from build123d import *

# Parameters (mm, degrees)
BOSS_EXTRUDE1_DEPTH      = 10
BOSS_EXTRUDE1_DEPTH_BACK = 0.01
SKETCH3_W                = 38
SKETCH3_H                = 54
CUT_EXTRUDE1_DEPTH       = 3
SKETCH5_W                = 38
SKETCH5_H                = 54
CUT_EXTRUDE3_DEPTH       = 3
SKETCH7_W                = 169
SKETCH7_H                = 58
CUT_EXTRUDE4_DEPTH       = 261.116514656
SKETCH15_W               = 20
SKETCH15_H               = 50
BOSS_EXTRUDE3_DEPTH      = 20.3
SKETCH18_W               = 47.4
SKETCH18_H               = 47.4
CUT_EXTRUDE18_DEPTH      = 261.715344958
SKETCH21_R               = 9
CUT_EXTRUDE21_DEPTH      = 20
SKETCH28_W               = 4.75290021
SKETCH28_H               = 9.947843747
BOSS_EXTRUDE6_DEPTH      = 115.870057685
SKETCH30_W               = 14.12
SKETCH30_H               = 25
CUT_EXTRUDE25_DEPTH      = 4.5
SKETCH33_R               = 1.55
CUT_EXTRUDE26_DEPTH      = 10.01
SKETCH36_W               = 38
SKETCH36_H               = 2
BOSS_EXTRUDE7_DEPTH      = 37
SKETCH39_R               = 6
SKETCH39_R_2             = 1.55
CUT_EXTRUDE28_DEPTH      = 2
SKETCH42_R               = 6
SKETCH42_R_2             = 1.55
CUT_EXTRUDE29_DEPTH      = 2


with BuildPart() as part:
    # Sketch1 → Boss-Extrude1 (new, two sides: drawn at the far end of the back side and taken through both)
    with BuildSketch(Plane.XY.offset(-BOSS_EXTRUDE1_DEPTH_BACK)):
        with BuildLine():
            Line((0, 0), (0, -37))
            Line((0, -37), (60, -37))
            Line((60, -37), (60, -52))
            Line((60, -52), (33.129942315, -78.870057685))
            Line((33.129942315, -78.870057685), (-55.850057685, -78.870057685))
            ThreePointArc((-55.850057685, -78.870057685), (-169.614041234, -90.257166815), (-239.999947532, -0.158696229))
            ThreePointArc((-239.999947532, -0.158696229), (-169.748285548, 90.207490359), (-55.850057685, 78.870057685))
            Line((-55.850057685, 78.870057685), (33.129942315, 78.870057685))
            Line((33.129942315, 78.870057685), (60, 52))
            Line((60, 52), (60, 37))
            Line((60, 37), (0, 37))
            Line((0, 37), (0, 0))
        make_face()
    extrude(amount=BOSS_EXTRUDE1_DEPTH + BOSS_EXTRUDE1_DEPTH_BACK)

    # Sketch3 → Cut-Extrude1 (cut)
    with BuildSketch(Plane.XY.offset(10)):
        with Locations((-19, 51.870057685)):
            Rectangle(SKETCH3_W, SKETCH3_H)
    extrude(amount=-CUT_EXTRUDE1_DEPTH, mode=Mode.SUBTRACT)

    # Sketch5 → Cut-Extrude3 (cut)
    with BuildSketch(Plane.XY.offset(10)):
        with Locations((-19, -51.870057685)):
            Rectangle(SKETCH5_W, SKETCH5_H)
    extrude(amount=-CUT_EXTRUDE3_DEPTH, mode=Mode.SUBTRACT)

    # Sketch7 → Cut-Extrude4 (cut, through all)
    with BuildSketch(Plane.XY.offset(10)):
        with Locations((-128.91309413, -19.94383898)):
            Rectangle(SKETCH7_W, SKETCH7_H)
    extrude(amount=-CUT_EXTRUDE4_DEPTH, mode=Mode.SUBTRACT)

    # Sketch15 → Boss-Extrude3 (add)
    with BuildSketch(Plane.XY.offset(10)):
        with Locations((-10, 0.20156489)):
            Rectangle(SKETCH15_W, SKETCH15_H)
    extrude(amount=BOSS_EXTRUDE3_DEPTH)

    # Sketch18 → Cut-Extrude18 (cut, through all)
    with BuildSketch(Plane.XY.offset(10)):
        with Locations((-80.42454895, 45.3)):
            Rectangle(SKETCH18_W, SKETCH18_H)
    extrude(amount=-CUT_EXTRUDE18_DEPTH, mode=Mode.SUBTRACT)

    # Sketch21 → Cut-Extrude21 (cut)
    with BuildSketch(Plane(origin=(0, 0, 0), x_dir=(0, 0, -1), z_dir=(1, 0, 0))):
        with Locations((-19.36187505, 12.37175029)):
            Circle(SKETCH21_R)
        with Locations((-19.26539558, -14.62824971)):
            Circle(SKETCH21_R)
        with BuildLine():
            Line((-9.491579533, 2.276446619), (-9.557448357, -4.178698144))
            ThreePointArc((-9.557448357, -4.178698144), (-12.081396215, -6.651657156), (-14.554355227, -4.127709299))
            Line((-14.554355227, -4.127709299), (-14.488486403, 2.327435464))
            ThreePointArc((-14.488486403, 2.327435464), (-11.964538545, 4.800394476), (-9.491579533, 2.276446619))
        make_face()
    extrude(amount=-CUT_EXTRUDE21_DEPTH, mode=Mode.SUBTRACT)

    # Sketch28 → Boss-Extrude6 (add)
    with BuildSketch(Plane.XZ.offset(78.870057685)):
        with Locations((16.603067585, 5.033719824)):
            Rectangle(SKETCH28_W, SKETCH28_H)
    extrude(amount=-BOSS_EXTRUDE6_DEPTH)

    # Sketch30 → Cut-Extrude25 (cut)
    with BuildSketch(Plane(origin=(0, 0, -0.01), x_dir=(-1, 0, 0), z_dir=(0, 0, -1))):
        with Locations((-7.06, -49.5)):
            Rectangle(SKETCH30_W, SKETCH30_H)
        Polygon((-14.38072485, 61.935396467), (-14.275539526, 36.935617747), (-0.155664505, 36.995026418), (-0.260849829, 61.994805138), align=None)
    extrude(amount=-CUT_EXTRUDE25_DEPTH, mode=Mode.SUBTRACT)

    # Sketch33 → Cut-Extrude26 (cut)
    with BuildSketch(Plane(origin=(0, 0, -0.01), x_dir=(-1, 0, 0), z_dir=(0, 0, -1))):
        with Locations((-7.06, -53.4)):
            Circle(SKETCH33_R)
        with Locations((-7.06, -49.4)):
            Circle(SKETCH33_R)
        with Locations((-7.06, -45.4)):
            Circle(SKETCH33_R)
        with Locations((-7.06, -41.4)):
            Circle(SKETCH33_R)
        with Locations((-7.228632788, 41.370889137)):
            Circle(SKETCH33_R)
        with Locations((-7.244931474, 45.370855931)):
            Circle(SKETCH33_R)
        with Locations((-7.261230159, 49.370822725)):
            Circle(SKETCH33_R)
        with Locations((-7.277528845, 53.370789519)):
            Circle(SKETCH33_R)
    extrude(amount=-CUT_EXTRUDE26_DEPTH, mode=Mode.SUBTRACT)

    # Sketch36 → Boss-Extrude7 (add)
    with BuildSketch(Plane.XY.offset(7)):
        Polygon((0.279518574, 78.814629504), (0.272425555, 76.814642082), (-37.727335467, 76.949409435), (-37.720242449, 78.949396858), align=None)
        with Locations((-19, -77.815125164)):
            Rectangle(SKETCH36_W, SKETCH36_H)
    extrude(amount=BOSS_EXTRUDE7_DEPTH)

    # Sketch39 → Cut-Extrude28 (cut)
    with BuildSketch(Plane.XZ.offset(78.815125164)):
        with Locations(Location((-19, 19, 0), (0, 0, 270))):
            Circle(SKETCH39_R)
        with Locations(Location((-34.499611559, 25.01055106, 0), (0, 0, 270))):
            Circle(SKETCH39_R_2)
        with Locations(Location((-3.563871147, 24.988758691, 0), (0, 0, 270))):
            Circle(SKETCH39_R_2)
        with Locations(Location((-28.819186805, 37.01055106, 0), (0, 0, 270))):
            Circle(SKETCH39_R_2)
        with Locations(Location((-9.177448314, 36.988758691, 0), (0, 0, 270))):
            Circle(SKETCH39_R_2)
        with Locations(Location((-28.819994175, 13.01055106, 0), (0, 0, 270))):
            Circle(SKETCH39_R_2)
        with Locations(Location((-9.230494356, 12.988758691, 0), (0, 0, 270))):
            Circle(SKETCH39_R_2)
    extrude(amount=-CUT_EXTRUDE28_DEPTH, mode=Mode.SUBTRACT)

    # Sketch42 → Cut-Extrude29 (cut)
    with BuildSketch(Plane(origin=(0.279518574, 78.814629504, 0), x_dir=(0.9999937111161443, -0.003546509292438372, 0), z_dir=(0.003546509292438372, 0.9999937111161443, 0))):
        with Locations(Location((-19.279713392, -19, 0), (0, 0, 180))):
            Circle(SKETCH42_R)
        with Locations(Location((-29.070149337, -13, 0), (0, 0, 180))):
            Circle(SKETCH42_R_2)
        with Locations(Location((-3.778432466, -25, 0), (0, 0, 180))):
            Circle(SKETCH42_R_2)
        with Locations(Location((-9.464104196, -13, 0), (0, 0, 180))):
            Circle(SKETCH42_R_2)
        with Locations(Location((-34.772326096, -25, 0), (0, 0, 180))):
            Circle(SKETCH42_R_2)
        with Locations(Location((-29.096493177, -37, 0), (0, 0, 180))):
            Circle(SKETCH42_R_2)
        with Locations(Location((-9.473371075, -37, 0), (0, 0, 180))):
            Circle(SKETCH42_R_2)
    extrude(amount=-CUT_EXTRUDE29_DEPTH, mode=Mode.SUBTRACT)


solid = part.part
The listing builds one solid part. Answer for the finished solid, in the listing's coordinates (mm). A direction names the side the tool comes from. Coordinates: 2 decimals unless noted, no trailing zeros. Loops run counter-clockwise (first coordinate to the right, second up) from the corner with the lowest first, then second, coordinate; pieces in that order, holes last. Notation, with made-up numbers: (-17.5, 13.25) -> (41.5, 13.25) arc R14 cw to (41.5, 24.25) -> close; hole circle Ø5 at (-20.5, 7.5). An arc over 180 degrees is marked (long way). Answer in a Markdown table with one row per item. Add a question column.
1. Flat-ended cylindrical pins translate along their axes: P1, Ø2, axis at y = -72, z = 13, coming from the -X side; P2, Ø3.5, axis at x = 7, z = 2.5, coming from the +Y side; P3, Ø6, axis at x = -9.5, y = -5, coming from the +Z side; P4, Ø8, axis at x = -166, z = 7.5, coming from the +Y side. Find the tip coordinate at first contact, or state that the pin passes through.
2. For faces 1 (the cylindrical face through (-14.94, -77.83, 23.42)), 2 (the flat face through (9, 50, 4.49)), 3 (the flat face through (-81, 21.6, 5)), 4 (the flat face through (-19, -50, 7)), determine the directions among +Z, -Z, +X, -X, +Y, -Y from which every point of the face is accessible in a straight line to the end or side of a thin tool.
3. Determine the mould class of faces 5 (the flat face through (7, -58, 10)), 6 (the cylindrical face through (-168.073, -90.903, 4.925)), 7 (the flat face through (-130, 9.056, 5)) for opening direction X: +X half, -X half, draft (parallel to the pull), parting line (faces both ways), or undercut.
4. The part is cut by section B-B, the plane z = 19. Write down the section's boundary in (x, y), then the cut area to 3 significant figures.
5. The part is cut by section D-D, the plane y = -19. Write down the section's boundary in (x, z), then the cut area to 3 significant figures.
6. Consider line 1 (X direction, y = -5, z = 9); line 2 (X direction, y = 4, z = 14); line 3 (Z direction, x = -105.5, y = 85). Determine where each line is inside the solid, lowest interval first. Write a range as [from, to].
7. The part is cut by section A-A, the plane x = -72.5. Write down the section's boundary in (y, z).
8. The part is cut by section C-C, the plane x = -202.5. Write down the section's boundary in (y, z).
Answer below:
| question | item | result |
|---|---|---|
| 1 | P1 | through |
| 1 | P2 | y = 78.87 |
| 1 | P3 | z = 30.3 |
| 1 | P4 | y = 93.22 |
| 2 | face 1 | -Y |
| 2 | face 2 | -Z |
| 2 | face 3 | +Z, -Z |
| 2 | face 4 | +Z |
| 3 | face 5 | draft |
| 3 | face 6 | parting line |
| 3 | face 7 | undercut |
| 4 | outline | (-38, -78.82) -> (-25, -78.82) -> (-25, -76.82) -> (-38, -76.82) -> close; (-37.73, 76.95) -> (-25.01, 76.9) -> (-25, 78.9) -> (-37.72, 78.95) -> close; (-20, -24.8) -> (0, -24.8) -> (0, -23.62) -> (-20, -23.62) -> close; (-20, -5.63) -> (0, -5.63) -> (0, 3.38) -> (-20, 3.38) -> close; (-20, 21.36) -> (0, 21.36) -> (0, 25.2) -> (-20, 25.2) -> close; (-13.01, 76.86) -> (0.27, 76.81) -> (0.28, 78.81) -> (-13, 78.86) -> close; (-13, -78.82) -> (0, -78.82) -> (0, -76.82) -> (-13, -76.82) -> close |
| 4 | area | 384 mm2 |
| 5 | outline | (-235.36, -0.01) -> (-213.41, -0.01) -> (-213.41, 10) -> (-235.36, 10) -> close; (-44.41, -0.01) -> (0, -0.01) -> (0, 11.4) -> (-20, 11.4) -> (-20, 10) -> (-44.41, 10) -> close; (-20, 27.13) -> (0, 27.13) -> (0, 30.3) -> (-20, 30.3) -> close; (14.23, 0.06) -> (18.98, 0.06) -> (18.98, 10.01) -> (14.23, 10.01) -> close |
| 5 | area | 803 mm2 |
| 6 | line 1 | [-239.12, -213.41], [-44.41, 0], [14.23, 18.98] |
| 6 | line 2 | [-20, 0] |
| 6 | line 3 | [-0.01, 10] |
| 7 | outline | (-88.45, -0.01) -> (-48.94, -0.01) -> (-48.94, 10) -> (-88.45, 10) -> close; (9.06, -0.01) -> (21.6, -0.01) -> (21.6, 10) -> (9.06, 10) -> close; (69, -0.01) -> (88.46, -0.01) -> (88.46, 10) -> (69, 10) -> close |
| 8 | outline | (-69.2, -0.01) -> (-48.94, -0.01) -> (-48.94, 10) -> (-69.2, 10) -> close; (9.06, -0.01) -> (69.19, -0.01) -> (69.19, 10) -> (9.06, 10) -> close |
